Read the model definition and answer for the solid it produces. Units are mm, in the model's axes. Give positions to 0.01 mm unless a question says otherwise; leave off trailing zeros. Order: outer loops, then holes, each group sorted by start corner. A loop starts at its lowest first (then second) coordinate and runs counter-clockwise, first axis right, second up.
Item 1: A cutting plane is placed at B-B (y = 0.65). Write down the section's boundary in (x, z), plus the area to 3 significant figures.
Item 2: Given pin 1 Ø3.5 at (x, z) = (-30.59, 0) entering from +Y, flat-ended and moving along its own axis, determine where the tip first touches the part or whether it passes through.
Item 3: A cutting plane is placed at A-A (z = 0). Write down the section's boundary in (x, y), plus the area to 3 significant figures.
Item 4: A cutting plane is placed at C-C (z = 4.25). Write down the section's boundary in (x, y).
Item 5: Find the intervals of material crossed by line 1 along X through (y, z) = (1.4, 0.75); line 2 along Z through (x, y) = (18.5, 1.5); line 3 along Z through (x, y) = (19, 0.55), in increasing order.
from build123d import *

# Parameters (mm, degrees)
SKETCH1_W             = 70
SKETCH1_H             = 10
BOSS_EXTRUDE1_DEPTH   = 2
F_5_0MM_DOWEL_HOLE1_D = 5
F_3_0MM_DOWEL_HOLE1_D = 3
SKETCH2_R             = 1.3
CUT_EXTRUDE1_DEPTH    = 3
FILLET1_R             = 3


with BuildPart() as part:
    # Sketch1 → Boss-Extrude1 (new body)
    with BuildSketch(Plane(origin=(0, 0, 0), x_dir=(1, 0, 0), z_dir=(0, 1, 0))):
        Rectangle(SKETCH1_W, SKETCH1_H)
    extrude(amount=BOSS_EXTRUDE1_DEPTH)

    # Ø5.0mm Dowel Hole1 (through all)
    with Locations(Plane(origin=(0, 2, 0), x_dir=(1, 0, 0), z_dir=(0, 1, 0))):
        with Locations((24.413883152, 0)):
            Hole(F_5_0MM_DOWEL_HOLE1_D / 2)

    # Ø3.0mm Dowel Hole1 (through all)
    with Locations(Plane(origin=(0, 2, 0), x_dir=(1, 0, 0), z_dir=(0, 1, 0))):
        with Locations((-30.586116848, 0)):
            Hole(F_3_0MM_DOWEL_HOLE1_D / 2)

    # Sketch2 → Cut-Extrude1 (cut)
    with BuildSketch(Plane(origin=(0, 2, 0), x_dir=(1, 0, 0), z_dir=(0, 1, 0))):
        with Locations((30.863883152, 0)):
            Circle(SKETCH2_R)
        with Locations((17.963883152, 0)):
            Circle(SKETCH2_R)
    extrude(amount=-CUT_EXTRUDE1_DEPTH, mode=Mode.SUBTRACT)

    # Fillet1
    fillet1_edges = [part.edges().sort_by_distance(p)[0] for p in [
        (35, 1, 5),
        (-35, 1, 5),
        (-35, 1, -5),
        (35, 1, -5),
    ]]
    fillet(fillet1_edges, radius=FILLET1_R)


solid = part.part
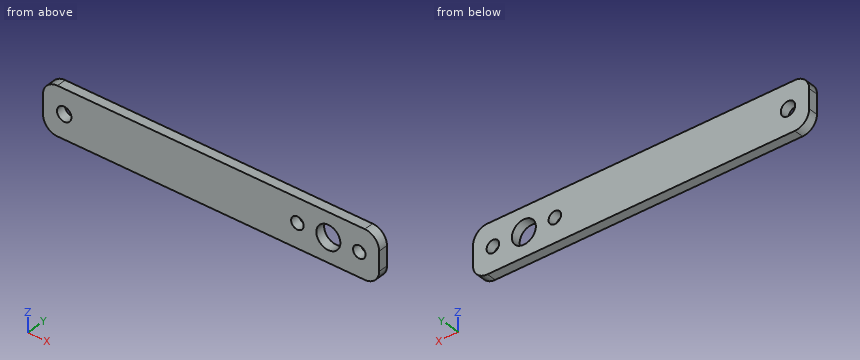
Response values:
1. outline: (-35, -2) arc R3 ccw to (-32, -5) - (32, -5) arc R3 ccw to (35, -2) - (35, 2) arc R3 ccw to (32, 5) - (-32, 5) arc R3 ccw to (-35, 2) - close; hole circle Ø3 at (-30.59, 0); hole circle Ø2.6 at (17.96, 0); hole circle Ø5 at (24.41, 0); hole circle Ø2.6 at (30.86, 0)
1. area: 655 mm2
2. pin 1: stops at y = 2
3. outline: (-35, 0) - (-32.09, 0) - (-32.09, 2) - (-35, 2) - close; (-29.09, 0) - (16.66, 0) - (16.66, 2) - (-29.09, 2) - close; (19.26, 0) - (21.91, 0) - (21.91, 2) - (19.26, 2) - close; (26.91, 0) - (29.56, 0) - (29.56, 2) - (26.91, 2) - close; (32.16, 0) - (35, 0) - (35, 2) - (32.16, 2) - close
3. area: 114 mm2
4. outline: (-33.98, 0) - (33.98, 0) - (33.98, 2) - (-33.98, 2) - close
5. line 1: x = -35 to -31.89, -29.29 to 16.9, 19.03 to 22.03, 26.8 to 29.8, 31.93 to 35
5. line 2: z = -5 to -1.18, 1.18 to 5
5. line 3: z = -5 to -0.79, 0.79 to 5
